Design review of the part built by this model. Coordinates are the model's own, in mm. A direction names the side the tool comes from. Give positions to 0.01 mm unless a question says otherwise; leave off trailing zeros. Order: outer loops, then holes, each group sorted by start corner. A loop starts at its lowest first (then second) coordinate and runs counter-clockwise, first axis right, second up. Notation, with made-up numbers: (24.25, 74) -> (39.25, 74) arc R12 ccw to (39.25, 93) -> close; hole circle Ø8 at (54, 6.25). An arc over 180 degrees is marked (long way). Answer in a Markdown table with one row per item. Add a question column.
```python
from build123d import *

# Parameters (mm, degrees)
BOSS_EXTRUDE1_START = -60
BOSS_EXTRUDE1_DEPTH = 5.5


with BuildPart() as part:
    # Sketch1 → Revolve1 (revolve)
    with BuildSketch(Plane.XY, mode=Mode.PRIVATE) as revolve1_sk:
        with BuildLine():
            Line((-17.75, 0), (0, 0))
            Line((0, 0), (0, 82.5))
            Line((0, 82.5), (-3.4, 82.5))
            Line((-3.4, 82.5), (-4, 81.9))
            Line((-4, 81.9), (-4, 17))
            Line((-4, 17), (-18, 17))
            ThreePointArc((-18, 17), (-19.414213562, 16.414213562), (-20, 15))
            Line((-20, 15), (-20, 4))
            Line((-20, 4), (-17.75, 4))
            Line((-17.75, 4), (-17.75, 0))
        make_face()
    revolve(revolve1_sk.sketch.rotate(Axis((0, 86.625, 0), (0, -1, 0)), 270), axis=Axis((0, 86.625, 0), (0, -1, 0)))

    # Sketch2 → Boss-Extrude1 (add)
    with BuildSketch(Plane(origin=(0, 82.5, 0), x_dir=(0, 0, -1), z_dir=(0, 1, 0)).offset(BOSS_EXTRUDE1_START)):
        Polygon((6.5, -3.75277675), (6.5, 3.75277675), (0, 7.505553499), (-6.5, 3.75277675), (-6.5, -3.75277675), (0, -7.505553499), align=None)
    extrude(amount=-BOSS_EXTRUDE1_DEPTH)

    # Sketch3 → Cut-Revolve1 (revolve, cut)
    with BuildSketch(Plane.XY):
        Polygon((7.505553499, 22.5), (6.5, 22.5), (7.505553499, 21.919443416), align=None)
        Polygon((7.505553499, 17), (6.5, 17), (7.505553499, 17.580556584), align=None)
    revolve(axis=Axis((0, 86.625, 0), (0, -1, 0)), mode=Mode.SUBTRACT)


solid = part.part
```
1) Clearance check with flat-ended pins moving along their axes: P1, Ø3, axis at x = 0.5, y = 20, coming from the +Z side; P2, Ø5, axis at x = -11, z = -11, coming from the +Y side; P3, Ø5, axis at x = -3.5, y = 37, coming from the -Z side. State where each tip first meets the part, or that it passes through.
2) Mouldability with a two-part tool opening along Y and no side actions: class faces 1 (the face through (5.6, 19.8, 3.3)), 2 (the face through (3.443, 17.206, 5.929)), 3 (the face through (3.36, 22.36, -5.85)), 4 (the face through (-6.86, 17.21, 0.02)) as +Y half, -Y half, draft (parallel to the pull), parting line (faces both ways), or undercut.
3) Machinability: for faces 5 (the face through (-3, 22.5, -3)), 6 (the face through (-5.66, 19.79, 3.2)), 7 (the face through (15.747, 1.972, 8.191)), which of the approach directions +Z, -Z, +X, -X, +Y, -Y give a long, thin tool a straight path to every point of the face, cutting with its end or side? Answer none if there is none.
4) Add section B-B, the plane y = 69. Write out the cut boundary in (x, z), and give its area (3 significant figures).
5) Add section A-A, the plane y = 7. Write out the cut boundary in (x, z).
6) For L1, parallel to Y at x = -10, z = 10.5; L2, parallel to Y at x = -5.5, z = 0; L3, parallel to Z at x = -2, y = 31, list the stretches that pass through material, from the lowest coordinate up.
Verdict:
| question | item | result |
|---|---|---|
| 1 | P1 | stops at z = 6.5 |
| 1 | P2 | stops at y = 17 |
| 1 | P3 | stops at z = -3.87 |
| 2 | face 1 | draft |
| 2 | face 2 | undercut |
| 2 | face 3 | +Y half |
| 2 | face 4 | undercut |
| 3 | face 5 | +Y |
| 3 | face 6 | +Z, -X, +Y |
| 3 | face 7 | -Y |
| 4 | outline | circle Ø8 at (0, 0) |
| 4 | area | 50.3 mm2 |
| 5 | outline | circle Ø40 at (0, 0) |
| 6 | L1 | y = 0 to 17 |
| 6 | L2 | y = 0 to 22.5 |
| 6 | L3 | z = -3.46 to 3.46 |
